from build123d import *

# Parameters (mm, degrees)
F0_R     = 65
F1_DEPTH = 5
F2_R     = 65
F2_R_2   = 60
F3_DEPTH = 30
F4_R     = 20
F5_DEPTH = 120
F6_R     = 20
F7_SIZE  = 1


with BuildPart() as f1:
    # F0 (on Front) → F1 (new body)
    with BuildSketch(Plane.XZ):
        Circle(F0_R)
    extrude(amount=-F1_DEPTH)

    # F2 (on face) → F3 (join)
    with BuildSketch(Plane.XZ):
        Circle(F2_R)
        Circle(F2_R_2, mode=Mode.SUBTRACT)
    extrude(amount=F3_DEPTH)

    # F4 (on face) → F5 (join)
    with BuildSketch(Plane(origin=(0, 5, 0), x_dir=(-1, 0, 0), z_dir=(0, 1, 0))):
        Circle(F4_R)
    extrude(amount=F5_DEPTH)

    # F6
    f6_edges = [f1.edges().sort_by_distance(p)[0] for p in [
        (20, 125, 0),
    ]]
    fillet(f6_edges, radius=F6_R)

    # F7
    f7_edges = [f1.edges().sort_by_distance(p)[0] for p in [
        (-65, 5, 0),
        (-65, -30, 0),
        (-60, -30, 0),
    ]]
    chamfer(f7_edges, length=F7_SIZE)


solid = f1.part
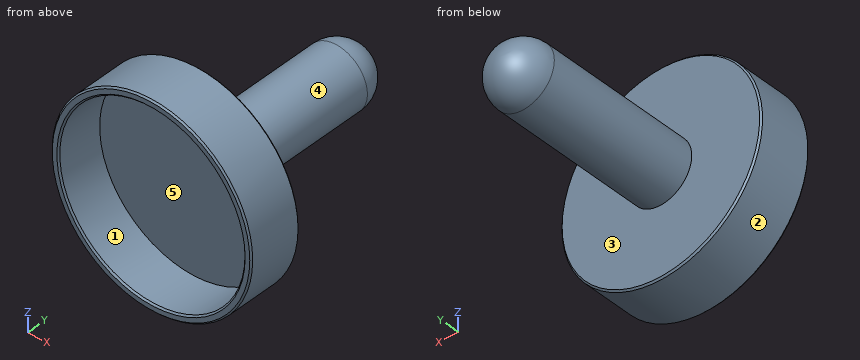
Read the model definition and answer for the solid it produces. Units are mm, in the model's axes. Face numbers are marked on the shaded views. A direction names the side the tool comes from. Coordinates: 2 decimals unless noted, no trailing zeros. Write each loop counter-clockwise with the first axis right and the second up, starting at its lowest first coordinate (ties: lowest second). Pieces come first, ordered by that corner, then holes. Notation, with made-up numbers: M 6.5,26.25 L 43.5,26.25 A11 ccw 43.5,30.25 Z; hole C 30,-15.75 d1. An arc over 180 degrees is marked long. Use a Markdown table: item, result.
Q1. Straight lines are drawn through the part: L1, parallel to Z at x = 0, y = -11.25; L2, parallel to Y at x = 18, z = -25; L3, parallel to Y at x = -33, z = 54. For each, find the intervals that lie inside material, in ascending order. Write a range as [from, to].
Answer block:
| item | result |
|---|---|
| L1 | z = [-65, -60], [60, 65] |
| L2 | y = [0, 5] |
| L3 | y = [-30, 5] |
Q2. The part is cut by section B-B, the plane x = 0. Write down the section's boundary in (y, z), then the cut area to 3 significant figures.
Answer block:
| item | result |
|---|---|
| outline | M -30,-64 L -29,-65 L 4,-65 L 5,-64 L 5,-20 L 105,-20 A20 ccw 105,20 L 5,20 L 5,64 L 4,65 L -29,65 L -30,64 L -30,61 L -29,60 L 0,60 L 0,-60 L -29,-60 L -30,-61 Z |
| area | 5,580 mm2 |
Q3. Which of the six approach directions +Z, -Z, +X, -X, +Y, -Y give full straight-line access (tool end or side, diameter ignored) to the marked faces 4 and 5?
Answer block:
| item | result |
|---|---|
| face 4 | +Y |
| face 5 | -Y |
Q4. The part is cut by section D-D, the plane y = 36.5. Write down the section's boundary in (x, z).
Answer block:
| item | result |
|---|---|
| outline | C 0,0 d40 |
Q5. Determine the mould class of the marked faces 1, 2 and 3 for opening direction Z: released by +Z, released by -Z, zero draft, split by the parting line, or undercut.
Answer block:
| item | result |
|---|---|
| face 1 | undercut |
| face 2 | split by the parting line |
| face 3 | zero draft |
Q6. The part is cut by section A-A, the plane z = 0. Write down the section's boundary in (x, y), then the cut area to 3 significant figures.
Answer block:
| item | result |
|---|---|
| outline | M -65,-29 L -64,-30 L -61,-30 L -60,-29 L -60,0 L 60,0 L 60,-29 L 61,-30 L 64,-30 L 65,-29 L 65,4 L 64,5 L 20,5 L 20,105 A20 ccw -20,105 L -20,5 L -64,5 L -65,4 Z |
| area | 5,580 mm2 |
Q7. Each of these flat-tipped pins is pushed along its axis until it touches: pin 1 Ø10 at (y, z) = (31, 16.5) entering from -X; pin 2 Ø6 at (x, z) = (-37.5, -17.5) entering from +Y; pin 3 Ø1.5 at (x, y) = (41, -9.5) entering from +Z. Where does it stop, or does it pass through?
Answer block:
| item | result |
|---|---|
| pin 1 | stops at x = -16.36 |
| pin 2 | stops at y = 5 |
| pin 3 | stops at z = 51.04 |
Q8. The part is cut by section C-C, the plane y = -11. Write down the section's boundary in (x, z), then the cut area to 3 significant figures.
Answer block:
| item | result |
|---|---|
| outline | C 0,0 d130; hole C 0,0 d120 |
| area | 1,960 mm2 |
